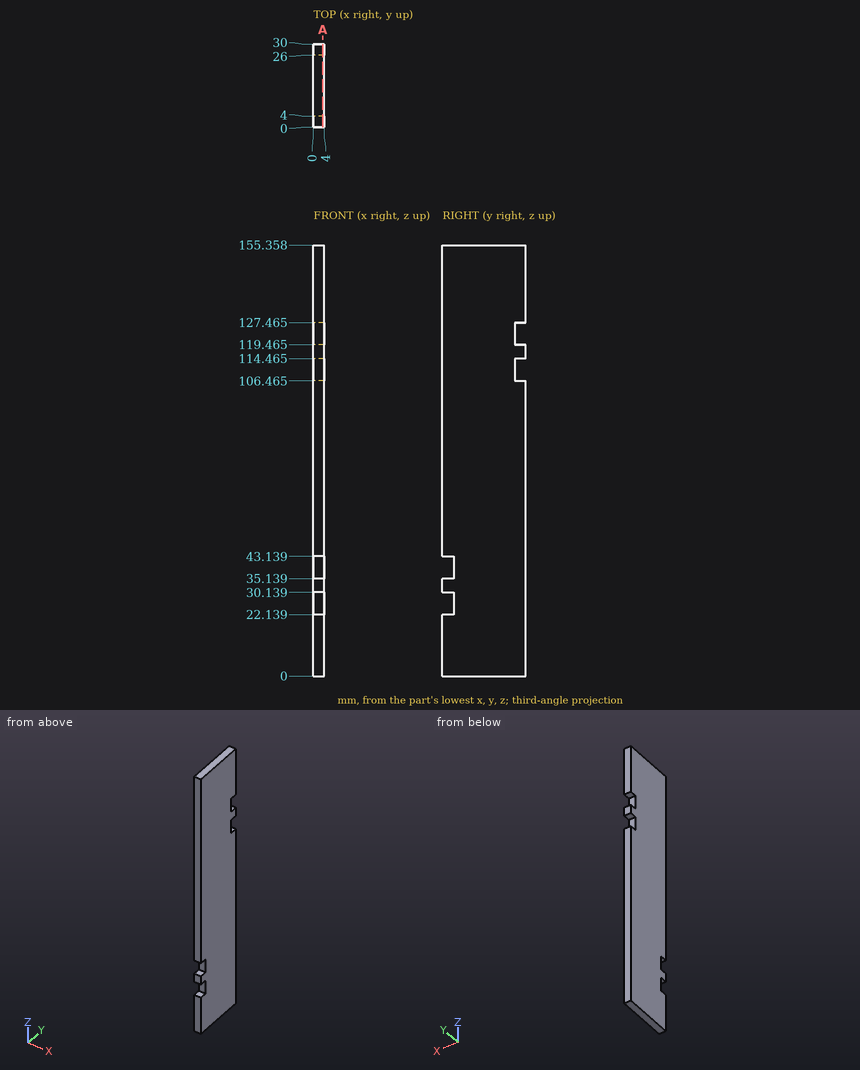
Input: dimensioned drawing with shaded views. Units: mm. Origin: part minimum x, y, z. Coordinates: 2 decimals unless noted, no trailing zeros. Order: outer loops, then holes, each group sorted by start corner. A loop starts at its lowest first (then second) coordinate and runs counter-clockwise, first axis right, second up. Notation, with made-up numbers: (46, -11.75) - (103, -11.75) arc R9 ccw to (103, -6.75) - close; hole circle Ø6 at (-34, 9). An arc over 180 degrees is marked (long way). Put each result on its own line as item: value.
1. Contact query for flat-ended pins moving along their axis: pin 1 Ø1.2 at (x, z) = (1.5, 38) entering from -Y; pin 2 Ø2 at (x, z) = (2, 123.5) entering from +Y. Output: stop coordinate, or through.
Report:
pin 1: stops at y = 4
pin 2: stops at y = 26
2. Cut plane A-A on x = 3.4. Return the cut outline in (y, z) (1 decimal).
Report:
outline: (0, 0) - (30, 0) - (30, 106.5) - (26, 106.5) - (26, 114.5) - (30, 114.5) - (30, 119.5) - (26, 119.5) - (26, 127.5) - (30, 127.5) - (30, 155.4) - (0, 155.4) - (0, 43.1) - (4, 43.1) - (4, 35.1) - (0, 35.1) - (0, 30.1) - (4, 30.1) - (4, 22.1) - (0, 22.1) - close
3. Line query: line 1 along Z through (x, y) = (0.2, 27.75) (1 decimal); line 2 along Z through (x, y) = (2.6, 2); line 3 along Y through (x, z) = (2, 113). Output: solid intervals per line, ascending.
Report:
line 1: z = 0 to 106.5, 114.5 to 119.5, 127.5 to 155.4
line 2: z = 0 to 22.14, 30.14 to 35.14, 43.14 to 155.36
line 3: y = 0 to 26
